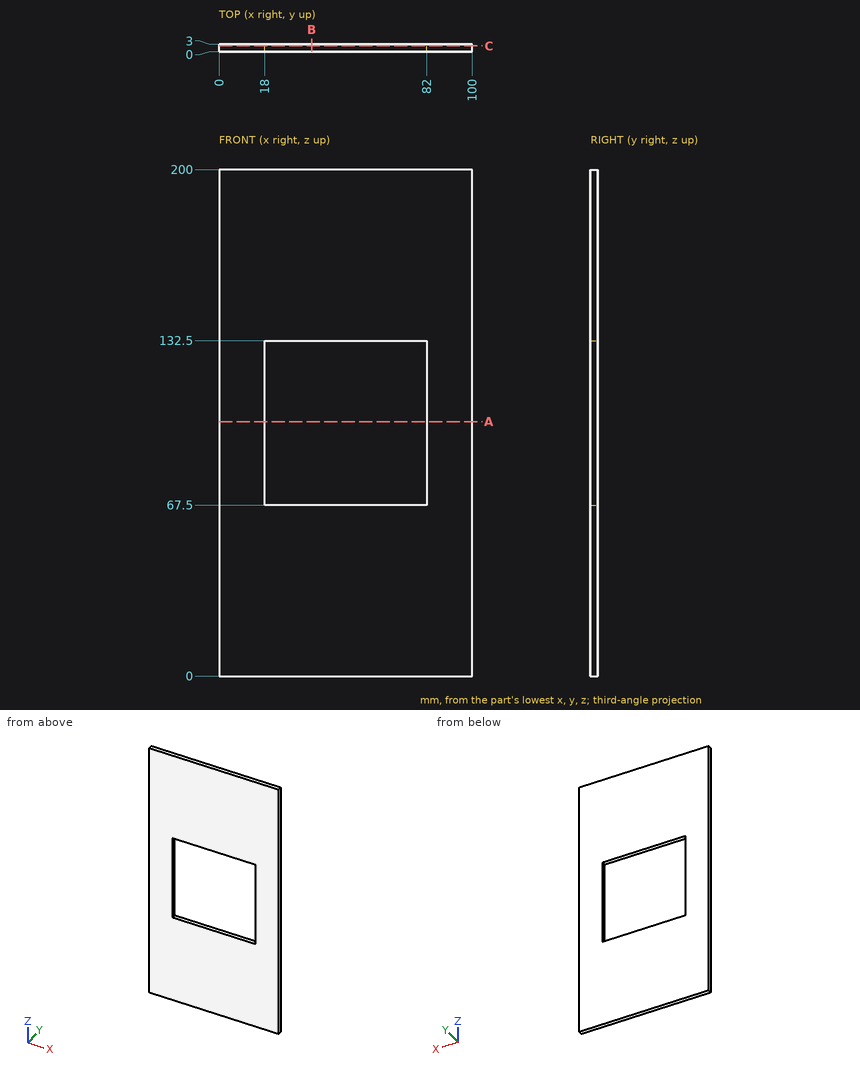
Print and shaded views of the part. All mm, measured from the part's lowest x, y and z. Round coordinates to 2 decimals unless told otherwise and drop trailing zeros. Write each loop counter-clockwise with the first axis right and the second up, starting at its lowest first coordinate (ties: lowest second). Pieces come first, ordered by that corner, then holes. Notation, with made-up numbers: (-11, 31.25) -> (8, 31.25) arc R21 ccw to (8, 50.25) -> close; hole circle Ø9 at (84, 25). An arc over 180 degrees is marked (long way). Return JSON: item names as keys, results as strings. Group by question number.
Q1. Probe L1, parallel to X at y = 0.3, z = 84; L2, parallel to Z at x = 62, y = 1.95. List the from-to ranges inside material, lowest first. Write a range as [from, to].
Q2. Saw through at A-A on z = 100.5. Write the cut outline in (x, y).
Q3. Saw through at B-B on x = 36.5. Write the cut outline in (y, z).
Q4. Saw through at C-C on y = 2.25. Write the cut outline in (x, z), plus the area to 3 significant figures.
Answer:
{
 "1": {"L1": "[0, 18], [82, 100]", "L2": "[0, 67.5], [132.5, 200]"},
 "2": {"outline": "(0, 0) -> (18, 0) -> (18, 3) -> (0, 3) -> close; (82, 0) -> (100, 0) -> (100, 3) -> (82, 3) -> close"},
 "3": {"outline": "(0, 0) -> (3, 0) -> (3, 67.5) -> (0, 67.5) -> close; (0, 132.5) -> (3, 132.5) -> (3, 200) -> (0, 200) -> close"},
 "4": {"outline": "(0, 0) -> (100, 0) -> (100, 200) -> (0, 200) -> close; hole (18, 67.5) -> (82, 67.5) -> (82, 132.5) -> (18, 132.5) -> close", "area": "15,800 mm2"}
}
